CAD build for the part. Positions are in the model's coordinates, mm. Round coordinates to 2 decimals unless told otherwise and drop trailing zeros. Write each loop counter-clockwise with the first axis right and the second up, starting at its lowest first coordinate (ties: lowest second). Pieces come first, ordered by that corner, then holes. Notation, with made-up numbers: (86.5, -4) - (114.5, -4) arc R23 cw to (114.5, 22) - close; hole circle Ø3 at (60.5, 19). An arc over 180 degrees is marked (long way). Put each result on its own line as item: value. Start each with the question number.
Item 1: Cut at B-B (x = 11.5). Give the cut face in (y, z), and give its area (3 significant figures).
Item 2: Drill centre lines: line 1 (Y direction, x = 0, z = -6.25); line 2 (X direction, y = 35.5, z = -3.5); line 3 (X direction, y = -38, z = -9.5). Where is each one in solid material? Low to high. Write a range as from..to.
Item 3: Cut at A-A (z = -7.75). Count the separate pieces of the cut face and the enclosed holes in it, and give its area (3 significant figures).
Item 4: Pin check, flat tips, straight feed: pin 1 Ø2.5 at (x, y) = (0, 36.5) entering from +Z; pin 2 Ø8 at (y, z) = (43, -8) entering from +X; pin 3 Ø4.5 at (x, y) = (-36.5, -36.5) entering from -Z; pin 4 Ø8 at (x, y) = (83, -23.5) entering from -Z. Stop position of each tip, or through.
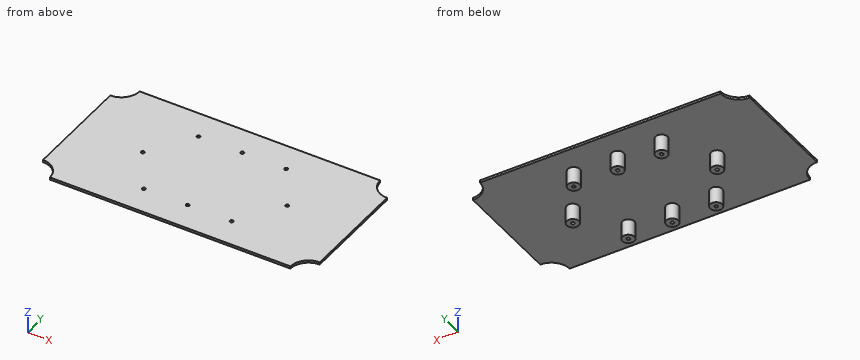
Autodesk Inventor part; units mm, degrees
ref_plane "YZ Plane" through (0, 0, 0) normal (1, 0, 0) x (0, 1, 0)
ref_plane "XZ Plane" through (0, 0, 0) normal (0, 1, 0) x (-1, 0, 0)
ref_plane "XY Plane" through (0, 0, 0) normal (0, 0, 1) x (1, 0, 0)
sketch "Skizze1" plane through (0, 0, 0) normal (0, 0, 1) x (1, 0, 0)
  line L0 (115, -60) -> (-115, -60)
  line L1 (-115, -60) -> (-115, 60)
  line L2 (-115, 60) -> (115, 60)
  line L3 (115, 60) -> (115, -60)
  line L4 (115, -60) -> (-115, 60) construction
  line L5 (-115, -60) -> (115, 60) construction
  circle A0 centre (-115, 60) radius 15
  circle A1 centre (115, 60) radius 15
  circle A2 centre (115, -60) radius 15
  circle A3 centre (-115, -60) radius 15
  point P0 (0, 0)
  point P1 (-115, -45)
  point P2 (-100, -60)
  point P3 (100, -60)
  point P4 (115, -45)
  point P5 (115, 45)
  point P6 (100, 60)
  point P7 (-100, 60)
  point P8 (-115, 45)
  dimension "d0" = 230
  dimension "d1" = 120
  dimension "d2" = 30
  dimension "d3" = 30
  dimension "d4" = 30
  dimension "d5" = 30
extrude "Extrusion1" add sketch "Skizze1" along normal blind 2 contours A3 L1 A0 L2 A1 L3 A2 L0
sketch "Skizze2" plane through (0, 0, 2) normal (0, 0, 1) x (1, 0, 0)
  line L0 (36.5, -36.5) -> (-36.5, -36.5)
  line L1 (-36.5, -36.5) -> (-36.5, 36.5)
  line L2 (-36.5, 36.5) -> (36.5, 36.5)
  line L3 (36.5, 36.5) -> (36.5, -36.5)
  line L4 (36.5, -36.5) -> (-36.5, 36.5) construction
  line L5 (-36.5, -36.5) -> (36.5, 36.5) construction
  point P0 (0, 0)
  point P1 (0, 36.5)
  point P2 (0, -36.5)
  point P3 (60, 0)
  point P4 (-60, 0)
  dimension "d8" = 73
  dimension "d9" = 73
  dimension "d25" = 23.5
  dimension "d26" = 23.5
hole "Bohrung1" at (0, 36.5, 2) at (0, -36.5, 2) at (-36.5, -36.5, 2) at (-36.5, 36.5, 2) at (36.5, 36.5, 2) at (36.5, -36.5, 2) at (-60, 0, 2) at (60, 0, 2) direction (0, 0, -1) diameter 2.8 end through all
sketch "Skizze3" plane through (0, 0, 0) normal (0, 0, -1) x (-1, 0, 0)
  circle A0 centre (-36.5, -36.5) radius 1.4
  circle A1 centre (-36.5, 36.5) radius 1.4
  circle A2 centre (36.5, 36.5) radius 1.4
  circle A3 centre (36.5, -36.5) radius 1.4
  circle A4 centre (0, -36.5) radius 1.4
  circle A5 centre (0, 36.5) radius 1.4
  line L0 (100, -60) -> (-100, -60)
  arc A6 (115, -45) -> (100, -60) centre (115, -60) ccw
  line L1 (115, 45) -> (115, -45)
  arc A7 (100, 60) -> (115, 45) centre (115, 60) ccw
  line L2 (-100, 60) -> (100, 60)
  arc A8 (-115, 45) -> (-100, 60) centre (-115, 60) ccw
  line L3 (-115, -45) -> (-115, 45)
  arc A9 (-100, -60) -> (-115, -45) centre (-115, -60) ccw
  circle A10 centre (36.5, -36.5) radius 5
  circle A11 centre (0, -36.5) radius 5
  circle A12 centre (-36.5, -36.5) radius 5
  circle A13 centre (-36.5, 36.5) radius 5
  circle A14 centre (0, 36.5) radius 5
  circle A15 centre (36.5, 36.5) radius 5
  circle A16 centre (-60, 0) radius 1.4
  circle A17 centre (60, 0) radius 1.4
  circle A18 centre (-36.5, -36.5) radius 1.4
  circle A19 centre (-36.5, 36.5) radius 1.4
  circle A20 centre (36.5, 36.5) radius 1.4
  circle A21 centre (36.5, -36.5) radius 1.4
  circle A22 centre (0, -36.5) radius 1.4
  circle A23 centre (0, 36.5) radius 1.4
  line L4 (100, -60) -> (-100, -60)
  arc A24 (115, -45) -> (100, -60) centre (115, -60) ccw
  line L5 (115, 45) -> (115, -45)
  arc A25 (100, 60) -> (115, 45) centre (115, 60) ccw
  line L6 (-100, 60) -> (100, 60)
  arc A26 (-115, 45) -> (-100, 60) centre (-115, 60) ccw
  line L7 (-115, -45) -> (-115, 45)
  arc A27 (-100, -60) -> (-115, -45) centre (-115, -60) ccw
  circle A28 centre (60, 0) radius 5
  circle A29 centre (-60, 0) radius 5
  point P0 (0, 0)
  dimension "d17" = 10
  dimension "d18" = 10
  dimension "d19" = 10
  dimension "d20" = 10
  dimension "d21" = 10
  dimension "d22" = 10
  dimension "d27" = 10
  dimension "d28" = 10
extrude "Extrusion2" add sketch "Skizze3" along normal blind 13.5 contours A10 | A11 | A12 | A13 | A14 | A15 | A28 | A29
ref_plane "Arbeitsebene1" through (-100, 0, 0) normal (0, 1, 0) x (1, 0, 0)
ref_plane "Arbeitsebene2" through (0, -45, 0) normal (-1, 0, 0) x (0, 0, 1)
properties part number "00_ElectroWallbox_Tpelectric_130x220x140_IP67_Inlet"
Output values:
1. outline: (-60, 0) - (60, 0) - (60, 2) - (-60, 2) - close
1. area: 240 mm2
2. line 1: -41.5..-37.9, -35.1..-31.5, 31.5..35.1, 37.9..41.5
2. line 2: -41.4..-37.48, -35.52..-31.6, -4.9..-0.98, 0.98..4.9, 31.6..35.52, 37.48..41.4
2. line 3: -41.27..-31.73, -4.77..4.77, 31.73..41.27
3. separate pieces: 8
3. enclosed holes: 8
3. area: 579 mm2
4. pin 1: through
4. pin 2: x = 40.83
4. pin 3: z = -13.5
4. pin 4: z = 0
